```python
from build123d import *

# Parameters (mm, degrees)
SKETCH1_R           = 12.7
BOSS_EXTRUDE1_DEPTH = 88.9
CUT_EXTRUDE1_DEPTH  = 169.930467649
SKETCH3_W           = 38.1
SKETCH3_H           = 16.138601809
CUT_EXTRUDE2_DEPTH  = 254


with BuildPart() as part:
    # Sketch1 → Boss-Extrude1 (new body)
    with BuildSketch(Plane.XY):
        Polygon((-125.52, 46.92), (26.88, 46.92), (26.88, 72.32), (-62.02, 116.77), (-125.52, 116.77), align=None)
        with Locations((-87.42, 78.67)):
            Circle(SKETCH1_R, mode=Mode.SUBTRACT)
    extrude(amount=BOSS_EXTRUDE1_DEPTH)

    # Sketch2 → Cut-Extrude1 (cut, through all)
    with BuildSketch(Plane(origin=(0, 116.77, 0), x_dir=(1, 0, 0), z_dir=(0, 1, 0))):
        Polygon((26.88, -63.451430224), (-23.92, -88.9), (26.88, -88.9), align=None)
    extrude(amount=-CUT_EXTRUDE1_DEPTH, mode=Mode.SUBTRACT)

    # Sketch3 → Cut-Extrude2 (cut)
    with BuildSketch(Plane.ZY.offset(125.52)):
        with Locations((44.45, 108.700699095)):
            Rectangle(SKETCH3_W, SKETCH3_H)
    extrude(amount=-CUT_EXTRUDE2_DEPTH, mode=Mode.SUBTRACT)


solid = part.part
```
Geometry check sheet. Reference: the model listing, model coordinates, mm. A direction names the side the tool comes from. Round coordinates to 2 decimals unless told otherwise and drop trailing zeros. Loops run counter-clockwise (first coordinate to the right, second up) from the corner with the lowest first, then second, coordinate; pieces in that order, holes last. Notation, with made-up numbers: M 37,65.25 L 96,65.25 A34 ccw 96,100.25 Z; hole C 8.5,37.25 d9. An arc over 180 degrees is marked long. Return JSON: item names as keys, results as strings. Group by question number.
(1) Set-up check for faces 5 (the face through (-89, 109, 63.5)), 6 (the face through (-93, 116.77, 76)): record each of +Z, -Z, +X, -X, +Y, -Y from which the full face is reachable in a straight line by a thin tool's end or side.
(2) Scan lines: line 1 along Y through (x, z) = (-87, 45); line 2 along Y through (x, z) = (-87.42, 18); line 3 along X through (y, z) = (68, 17.5). Record each from-to range of solid material in increasing order. Write a range as [from, to].
(3) Section check A-A, the plane x = -87.42. Enter the section's corners in (y, z), and give its area (3 significant figures).
(4) Go/stop test with flat-tipped pins: pin 1 (4 mm diameter, centred on y = 103, z = 30.5, fed in from +X); pin 2 (19 mm diameter, centred on x = -101.5, z = 45.5, fed in from +Y); pin 3 (5 mm diameter, centred on x = 10, z = 55, fed in from +Y). Record where each tip stops, or that it passes through.
(5) Mould release check, pull along Z, two halves, no side actions. Record for faces 1 (the face through (1.836, 67.031, 75.998)), 2 (the face through (-67, 75, 0)), 3 (the face through (-89, 109, 25.4)), 4 (the face through (-78, 100.631, 44)): pulls with the +Z half, pulls with the -Z half, needs draft (parallel to the pull), parting line crosses it, or undercut.
(6) Section check D-D, the plane x = -114. Enter the section's corners in (y, z), and give its area (3 significant figures).
(7) Section check B-B, the plane z = 22. Enter the section's corners in (x, y), and give its area (3 significant figures).
(8) Section check C-C, the plane y = 78.67. Enter the section's corners in (x, z).
Data:
{
 "1": {"face 5": "+X, -X, +Y", "face 6": "+Z, -Z, +X, -X, +Y"},
 "2": {"line 1": "[46.92, 65.98], [91.36, 100.63]", "line 2": "[46.92, 65.97], [91.37, 116.77]", "line 3": "[-125.52, -94.31], [-80.53, 26.88]"},
 "3": {"outline": "M 46.92,0 L 65.97,0 L 65.97,88.9 L 46.92,88.9 Z; M 91.37,0 L 116.77,0 L 116.77,25.4 L 100.63,25.4 L 100.63,63.5 L 116.77,63.5 L 116.77,88.9 L 91.37,88.9 Z", "area": "3,340 mm²"},
 "4": {"pin 1": "through", "pin 2": "y = 100.63", "pin 3": "y = 82.01"},
 "5": {"face 1": "pulls with the +Z half", "face 2": "pulls with the -Z half", "face 3": "undercut", "face 4": "undercut"},
 "6": {"outline": "M 46.92,0 L 116.77,0 L 116.77,25.4 L 100.63,25.4 L 100.63,63.5 L 116.77,63.5 L 116.77,88.9 L 46.92,88.9 Z", "area": "5,590 mm²"},
 "7": {"outline": "M -125.52,46.92 L 26.88,46.92 L 26.88,72.32 L -62.02,116.77 L -125.52,116.77 Z; hole C -87.42,78.67 d25.4", "area": "8,160 mm²"},
 "8": {"outline": "M -125.52,0 L -100.12,0 L -100.12,88.9 L -125.52,88.9 Z; M -74.72,0 L 14.18,0 L 14.18,69.81 L -23.92,88.9 L -74.72,88.9 Z"}
}
